```python
from build123d import *

# Parameters (mm, degrees)
F0_R     = 25.4
F1_DEPTH = 12.7


with BuildPart() as f1:
    # F0 (on Top) → F1 (new body)
    with BuildSketch(Plane.XY):
        with BuildLine():
            ThreePointArc((152.210637, -7.594865), (152.352652, -3.798613), (152.4, 0))
            ThreePointArc((152.4, 0), (152.380736, 2.423103), (152.322947, 4.845593))
            ThreePointArc((152.322947, 4.845593), (141.912408, 13.707712), (150.434272, 24.398564))
            ThreePointArc((150.434272, 24.398564), (149.313035, 30.518479), (147.942937, 36.587529))
            ThreePointArc((147.942937, 36.587529), (135.909535, 43.077036), (142.007699, 55.313412))
            ThreePointArc((142.007699, 55.313412), (139.631639, 61.063618), (137.022854, 66.712049))
            ThreePointArc((137.022854, 66.712049), (123.898547, 70.542066), (127.30343, 83.783034))
            ThreePointArc((127.30343, 83.783034), (123.777584, 88.909334), (120.045438, 93.887448))
            ThreePointArc((120.045438, 93.887448), (106.410408, 94.888661), (106.971492, 108.548883))
            ThreePointArc((106.971492, 108.548883), (102.451727, 112.824659), (97.761205, 116.912389))
            ThreePointArc((97.761205, 116.912389), (84.218213, 115.040539), (81.910694, 128.51614))
            ThreePointArc((81.910694, 128.51614), (76.596814, 131.752374), (71.155269, 134.769016))
            ThreePointArc((71.155269, 134.769016), (58.303006, 130.10685), (53.228892, 142.802119))
            ThreePointArc((53.228892, 142.802119), (47.355806, 144.855748), (41.403792, 146.667945))
            ThreePointArc((41.403792, 146.667945), (29.810413, 139.421563), (22.194015, 150.775282))
            ThreePointArc((22.194015, 150.775282), (16.021353, 151.555522), (9.821987, 152.083163))
            ThreePointArc((9.821987, 152.083163), (0, 142.572904), (-9.821987, 152.083163))
            ThreePointArc((-9.821987, 152.083163), (-13.282535, 151.820072), (-16.736195, 151.478249))
            ThreePointArc((-16.736195, 151.478249), (-16.661745, 150.783242), (-16.636886, 150.084702))
            ThreePointArc((-16.636886, 150.084702), (-25.44977, 140.310082), (-36.081733, 148.067108))
            ThreePointArc((-36.081733, 148.067108), (-42.095292, 146.470974), (-48.038691, 144.630717))
            ThreePointArc((-48.038691, 144.630717), (-47.5856, 142.959149), (-47.43299, 141.233999))
            ThreePointArc((-47.43299, 141.233999), (-55.223917, 131.620163), (-66.243396, 137.250036))
            ThreePointArc((-66.243396, 137.250036), (-71.790301, 134.431814), (-77.217553, 131.389533))
            ThreePointArc((-77.217553, 131.389533), (-76.085391, 128.872443), (-75.697812, 126.139803))
            ThreePointArc((-75.697812, 126.139803), (-82.489349, 116.793296), (-93.476655, 120.365589))
            ThreePointArc((-93.476655, 120.365589), (-98.311696, 116.449862), (-102.98288, 112.340048))
            ThreePointArc((-102.98288, 112.340048), (-100.909017, 109.179225), (-100.181858, 105.469379))
            ThreePointArc((-100.181858, 105.469379), (-106.007645, 96.493782), (-116.577616, 98.160172))
            ThreePointArc((-116.577616, 98.160172), (-120.487052, 93.320043), (-124.19567, 88.324377))
            ThreePointArc((-124.19567, 88.324377), (-120.970356, 84.782436), (-119.802768, 80.136498))
            ThreePointArc((-119.802768, 80.136498), (-124.707149, 71.631282), (-134.525062, 71.615415))
            ThreePointArc((-134.525062, 71.615415), (-137.336068, 66.064849), (-139.918176, 60.404173))
            ThreePointArc((-139.918176, 60.404173), (-135.39715, 56.791586), (-133.693165, 51.261044))
            ThreePointArc((-133.693165, 51.261044), (-137.730696, 43.320467), (-146.525595, 41.904774))
            ThreePointArc((-146.525595, 41.904774), (-148.113906, 35.889145), (-149.455356, 29.813698))
            ThreePointArc((-149.455356, 29.813698), (-143.569406, 26.473362), (-141.239, 20.119508))
            ThreePointArc((-141.239, 20.119508), (-144.473844, 12.83157), (-152.048709, 10.341661))
            ThreePointArc((-152.048709, 10.341661), (-152.344113, 4.126898), (-152.385603, -2.094742))
            ThreePointArc((-152.385603, -2.094742), (-145.146605, -4.804697), (-142.106697, -11.911447))
            ThreePointArc((-142.106697, -11.911447), (-144.611911, -18.465977), (-150.850248, -21.678624))
            ThreePointArc((-150.850248, -21.678624), (-149.839684, -27.817785), (-148.579381, -33.910582))
            ThreePointArc((-148.579381, -33.910582), (-140.082526, -35.634948), (-136.257897, -43.415835))
            ThreePointArc((-136.257897, -43.415835), (-138.114625, -49.164318), (-142.98319, -52.740568))
            ThreePointArc((-142.98319, -52.740568), (-140.711332, -58.532735), (-138.20495, -64.227345))
            ThreePointArc((-138.20495, -64.227345), (-128.627028, -64.632158), (-123.951157, -73.000952))
            ThreePointArc((-123.951157, -73.000952), (-125.24773, -77.87968), (-128.795312, -81.471023))
            ThreePointArc((-128.795312, -81.471023), (-125.362592, -86.660144), (-121.72093, -91.704827))
            ThreePointArc((-121.72093, -91.704827), (-111.314719, -90.494981), (-105.730518, -99.358934))
            ThreePointArc((-105.730518, -99.358934), (-106.561474, -103.31384), (-108.913814, -106.599911))
            ThreePointArc((-108.913814, -106.599911), (-104.471982, -110.956591), (-99.856025, -115.128338))
            ThreePointArc((-99.856025, -115.128338), (-88.941006, -112.063704), (-82.401454, -121.324583))
            ThreePointArc((-82.401454, -121.324583), (-82.866492, -124.311837), (-84.217593, -127.016365))
            ThreePointArc((-84.217593, -127.016365), (-78.963006, -130.34801), (-73.576812, -133.462402))
            ThreePointArc((-73.576812, -133.462402), (-62.526605, -128.371697), (-54.995268, -137.926869))
            ThreePointArc((-54.995268, -137.926869), (-55.198142, -139.913365), (-55.798387, -141.817841))
            ThreePointArc((-55.798387, -141.817841), (-49.963335, -143.977169), (-44.045008, -145.896529))
            ThreePointArc((-44.045008, -145.896529), (-33.272061, -138.688287), (-24.723496, -148.431858))
            ThreePointArc((-24.723496, -148.431858), (-24.770866, -149.395581), (-24.912517, -150.350013))
            ThreePointArc((-24.912517, -150.350013), (-18.754947, -151.241568), (-12.566119, -151.881048))
            ThreePointArc((-12.566119, -151.881048), (-2.574032, -142.549666), (7.074654, -152.235703))
            ThreePointArc((7.074654, -152.235703), (13.282535, -151.820072), (19.468278, -151.151401))
            ThreePointArc((19.468278, -151.151401), (27.288417, -139.93704), (38.749078, -147.39155))
            ThreePointArc((38.749078, -147.39155), (44.73284, -145.687107), (50.642046, -143.739846))
            ThreePointArc((50.642046, -143.739846), (55.944534, -131.138255), (68.710532, -136.031698))
            ThreePointArc((68.710532, -136.031698), (74.205652, -133.11379), (79.577094, -129.974021))
            ThreePointArc((79.577094, -129.974021), (82.127527, -116.542276), (95.634518, -118.658329))
            ThreePointArc((95.634518, -118.658329), (100.398075, -114.655948), (104.994299, -110.46247))
            ThreePointArc((104.994299, -110.46247), (104.67993, -96.794345), (118.330814, -96.039463))
            ThreePointArc((118.330814, -96.039463), (122.152227, -91.129542), (125.770049, -86.067734))
            ThreePointArc((125.770049, -86.067734), (122.604775, -72.767451), (135.796091, -69.175007))
            ThreePointArc((135.796091, -69.175007), (138.506429, -63.574596), (140.985916, -57.868224))
            ThreePointArc((140.985916, -57.868224), (135.109664, -45.523746), (147.258268, -39.252549))
            ThreePointArc((147.258268, -39.252549), (148.737713, -33.209225), (149.969257, -27.11055))
            ThreePointArc((149.969257, -27.11055), (141.641797, -16.267586), (152.210637, -7.594865))
        make_face()
        Circle(F0_R, mode=Mode.SUBTRACT)
    extrude(amount=F1_DEPTH)


solid = f1.part
```
Here's how the part is built. I have some questions about the finished solid (model axes, mm). A direction names the side the tool comes from. Round coordinates to 2 decimals unless told otherwise and drop trailing zeros. Order: outer loops, then holes, each group sorted by start corner. A loop starts at its lowest first (then second) coordinate and runs counter-clockwise, first axis right, second up. Notation, with made-up numbers: M 68,79 L 78,79 A23 cw 78,97 Z; hole C 53,-24.5 d9. An arc over 180 degrees is marked long. Use CSV: the item, a comma, the result in double quotes.
1) I want a section at C-C (x = 57). List the corners of the cut face in (y, z) for me, then the cut area to 3 significant figures.
Taken from the geometry:
outline,"M -130.76,0 L 130.81,0 L 130.81,12.7 L -130.76,12.7 Z"
area,"3,320 mm^2"
2) If we mould it in two halves opening along X, with no side actions, what happens to faces 3 (the cylindrical face through (84.39, 114.92, 6.26)), 4 (the cylindrical face through (-79.04, -130.3, 6.26)), 5 (the cylindrical face through (102.516, 112.766, 6.261))? For each: pulls with the +X half, pulls with the -X half, needs draft (parallel to the pull), parting line crosses it, or undercut.
Taken from the geometry:
face 3,"undercut"
face 4,"pulls with the -X half"
face 5,"pulls with the +X half"
3) I want a section at B-B (x = 110.5). List the corners of the cut face in (y, z) for me, then the cut area to 3 significant figures.
Taken from the geometry:
outline,"M -93.74,0 L 92.15,0 L 92.15,12.7 L -93.74,12.7 Z"
area,"2,360 mm^2"
4) I need wall thicknesses on line 1 along Y through (x, z) = (0, 6); line 2 along X through (y, z) = (7, 10); line 3 along X through (y, z) = (106, 5). Which ranges of each line are inside material? Lowest first, please. Write a range as [from, to].
Taken from the geometry:
line 1,"[-142.94, -25.4], [25.4, 142.57]"
line 2,"[-152.24, -24.42], [24.42, 145.53]"
line 3,"[-100.2, 105.05]"
5) I want a section at A-A (x = 0). List the corners of the cut face in (y, z) for me.
Taken from the geometry:
outline,"M -142.94,0 L -25.4,0 L -25.4,12.7 L -142.94,12.7 Z; M 25.4,0 L 142.57,0 L 142.57,12.7 L 25.4,12.7 Z"
6) On a 3-axis mill with a long thin cutter (end or side, diameter ignored), from which of +Z, -Z, +X, -X, +Y, -Y can I reach the whole of each face in a straight line? I mean faces 1 (the cylindrical face through (74.13, -133.156, 6.261)), 2 (the cylindrical face through (-82.325, 116.848, 6.261)). Say none if no direction works.
Taken from the geometry:
face 1,"+Z, -Z, +X, -Y"
face 2,"+Z, -Z"
7) I'm going to push flat-ended pins straight in: P1, Ø2, axis at x = -67.5, z = 4, coming from the -Y side; P2, Ø5, axis at x = 103.5, z = 2, coming from the -Y side; P3, Ø2, axis at x = 28.5, z = 4, coming from the +Y side. Where does each tip first touch, or does it pass through?
Taken from the geometry:
P1,"y = -128.81"
P2,"y = -114.13"
P3,"y = 140.23"
